Autodesk Inventor part; units mm, degrees
ref_plane "YZ Plane" through (0, 0, 0) normal (1, 0, 0) x (0, 1, 0)
ref_plane "XZ Plane" through (0, 0, 0) normal (0, 1, 0) x (-1, 0, 0)
ref_plane "XY Plane" through (0, 0, 0) normal (0, 0, 1) x (1, 0, 0)
sketch "Sketch1" plane through (0, 0, 0) normal (0, 0, 1) x (1, 0, 0)
  line L0 (0, 0) -> (0, 6)
  line L1 (0, 6) -> (41.5, 6)
  line L2 (41.5, 6) -> (41.5, 23.5)
  line L3 (41.5, 23.5) -> (88, 23.5)
  line L4 (88, 23.5) -> (88, 17.5)
  line L5 (88, 17.5) -> (47.5, 17.5)
  line L6 (47.5, 17.5) -> (47.5, 0)
  line L7 (47.5, 0) -> (0, 0)
  dimension "d0" = 6
  dimension "d1" = 6
  dimension "d2" = 6
  dimension "d3" = 88
  dimension "d4" = 41.5
  dimension "d5" = 17.5
extrude "Extrusion1" add sketch "Sketch1" along normal blind 45
sketch "Sketch3" plane through (88, 17.5, 0) normal (0, -1, 0) x (1, 0, 0)
  line L0 (0, 0) -> (-40.5, 0)
  line L1 (-40.5, 0) -> (-40.5, 45)
  point P0 (-38, 0)
  point P1 (-88, 0)
  point P2 (-17.9956, 22.5044)
  dimension "d9" = 22.5044
  dimension "d10" = 22.5044
hole "Hole1" at (70.0044, 17.5, 22.5044) direction (0, 1, 0) diameter 9 end through all
sketch "Sketch4" plane through (0, 0, 0) normal (0, -1, 0) x (1, 0, 0)
  line L0 (47.5, 45) -> (0, 45)
  line L1 (47.5, 0) -> (47.5, 45)
  circle A0 centre (30, 22.4956) radius 4.5
  circle A1 centre (12, 22.4956) radius 4.5
  line L2 (30, 17.9956) -> (12, 17.9956)
  line L3 (12, 26.9956) -> (30, 26.9956)
  dimension "d18" = 17.5
  dimension "d19" = 18
  dimension "d20" = 22.5044
  dimension "d21" = 9
  dimension "d22" = 9
extrude "Extrusion2" cut sketch "Sketch4" against normal blind 45
fillet "Fillet2" radius 2.5 1 edges at (47.5, 17.5, 22.5)
fillet "Fillet3" radius 4 4 edges at (88, 23.5, 22.5) (41.5, 23.5, 22.5) (0, 6, 22.5) (41.5, 6, 22.5)
equation "\"d1\" = d0"
equation "\"d2\" = d0"
equation "\"d22\" = d21"
properties part number "093P45LN Bracket" material "Aluminum-6061"
CAD build for the part. Positions are in the model's coordinates, mm. A direction names the side the tool comes from. Give positions to 0.01 mm unless a question says otherwise; leave off trailing zeros. Write each loop counter-clockwise with the first axis right and the second up, starting at its lowest first coordinate (ties: lowest second). Pieces come first, ordered by that corner, then holes. Notation, with made-up numbers: M 33.5,-12 L 47.5,-12 A13 ccw 47.5,-1 Z; hole C 39,13 d3. An arc over 180 degrees is marked long. Return JSON: item names as keys, results as strings. Group by question number.
(1) Band-saw the part on D-D (x = 66.5). Give the cut face in (y, z), and give its area (3 significant figures).
(2) Mould opens along X. For faces 1 (the face through (64, 23.5, 22)), 2 (the face through (41.5, 15, 22)), 3 (the face through (34.5, 3, 22.4)) say: pulls with the +X half, pulls with the -X half, needs draft (parallel to the pull), parting line crosses it, or undercut.
(3) 3-axis set-ups, long thin cutter, end or side, ignore diameter. For faces 4 (the face through (21, 6, 17)), 5 (the face through (44, 12, 45)), 6 (the face through (47.5, 8, 22)), 7 (the face through (86.859, 22.297, 22.815)), 8 (the face through (21, 3, 17.996)): which of +Z, -Z, +X, -X, +Y, -Y reach the whole face in a straight line?
(4) Band-saw the part on A-A (x = 26.5). Give the cut face in (y, z).
(5) Flat gauge pins, fed straight in: pin 1 Ø2 at (y, z) = (14, 23.5) entering from -X; pin 2 Ø4.5 at (y, z) = (4.5, 11.5) entering from +X; pin 3 Ø2 at (x, y) = (75.5, 16) entering from +Z; pin 4 Ø10 at (y, z) = (11, 31) entering from +X. Where does each tip first touch, or does it go through?
(6) Drill centre lines: L1, parallel to Y at x = 22, z = 39; L2, parallel to Y at x = 82, z = 34.5; L3, parallel to X at y = 11.25, z = 12. Where is each one in solid material? Low to high. Write a range as [from, to].
(7) Band-saw the part on B-B (z = 8.5). Give the cut face in (x, y).
(8) Band-saw the part on C-C (y = 3.75). Give the cut face in (x, z).
Entries:
{
 "1": {"outline": "M 17.5,0 L 23.5,0 L 23.5,19.68 L 17.5,19.68 Z; M 17.5,25.33 L 23.5,25.33 L 23.5,45 L 17.5,45 Z", "area": "236 mm^2"},
 "2": {"face 1": "needs draft", "face 2": "pulls with the -X half", "face 3": "undercut"},
 "3": {"face 4": "+Z, -Z, -X, +Y", "face 5": "+Z, +X, -X, +Y, -Y", "face 6": "+Z, -Z, +X, -Y", "face 7": "+Z, -Z, +X, +Y", "face 8": "+Y, -Y"},
 "4": {"outline": "M 0,0 L 6,0 L 6,18 L 0,18 Z; M 0,27 L 6,27 L 6,45 L 0,45 Z"},
 "5": {"pin 1": "stops at x = 41.5", "pin 2": "stops at x = 47.5", "pin 3": "passes through", "pin 4": "stops at x = 47.71"},
 "6": {"L1": "y = [0, 6]", "L2": "y = [17.5, 23.5]", "L3": "x = [41.5, 47.5]"},
 "7": {"outline": "M 0,0 L 47.5,0 L 47.5,15 A2.5 cw 50,17.5 L 88,17.5 L 88,19.5 A4 ccw 84,23.5 L 45.5,23.5 A4 ccw 41.5,19.5 L 41.5,10 A4 cw 37.5,6 L 4,6 A4 ccw 0,2 Z"},
 "8": {"outline": "M 0.4,0 L 47.5,0 L 47.5,45 L 0.4,45 Z; hole M 12,18 L 30,18 A4.5 ccw 30,27 L 12,27 A4.5 ccw Z"}
}
